Can you work these out from the model? Positions are in its coordinate system, mm. Face numbers are marked on the shaded views. A direction names the side the tool comes from. Coordinates: 2 decimals unless noted, no trailing zeros. Order: outer loops, then holes, each group sorted by start corner. A loop starts at its lowest first (then second) coordinate and runs counter-clockwise, first axis right, second up. Notation, with made-up numbers: (86, -19) -> (107, -19) arc R9 ccw to (107, -7) -> close; hole circle Ø7 at (-3, 55.5). An arc over 180 degrees is marked (long way). Use a Markdown table: item, result. Add a question column.
1. We'd pull the mould along X, two halves only. Please class the marked faces 5, 6 and 7: pulls with the +X half, pulls with the -X half, needs draft (parallel to the pull), parting line crosses it, or undercut.
2. Suppose I cut it at D-D, the plane y = -7. List the corners of the cut face in (x, z) for me.
3. For pin 1 Ø5 at (x, z) = (-16.5, 24) entering from +Y; pin 2 Ø4 at (x, y) = (-22, -3.5) entering from -Z; pin 3 Ø3 at (y, z) = (-3.5, 19.5) entering from +X; pin 4 Ø2 at (x, z) = (-2.5, 21) entering from -Y, each with a flat end and sliding along its axis, tell me the tip position at first contact or that it passes through.
4. Suppose I cut it at C-C, the plane y = -2.25. List the corners of the cut face in (x, z) for me, then the cut area to 3 significant figures.
5. Suppose I cut it at B-B, the plane x = -17.5. List the corners of the cut face in (y, z) for me.
6. If I drill on line 1 along X through (y, z) = (-1.5, 17); line 2 along Y through (x, z) = (-23.5, 23.25); line 3 along X through (y, z) = (-7, 25.25), over which ranges is the centre line in solid material (lowest first)? Write a range as from..to.
7. For the marked faces 1, 2, 3 and 4, which set-ups out of +Z, -Z, +X, -X, +Y, -Y let a thin tool reach every point of the face, with its end or its side?
8. Suppose I cut it at A-A, the plane z = 27.75. List the corners of the cut face in (x, y) for me, then the cut area to 3 significant figures.
```python
from build123d import *

# Parameters (mm, degrees)
SKETCH1_W           = 35
SKETCH1_H           = 175
BOSS_EXTRUDE1_DEPTH = 7.5
SKETCH2_W           = 25
SKETCH2_H           = 6.5
CUT_EXTRUDE1_DEPTH  = 179.623206779
CUT_EXTRUDE2_DEPTH  = 179.623206779
SKETCH4_W           = 4
SKETCH4_H           = 6.5
CUT_EXTRUDE3_DEPTH  = 179.623206779
SKETCH5_W           = 4
SKETCH5_H           = 6.5
CUT_EXTRUDE4_DEPTH  = 179.623206779
CUT_EXTRUDE5_DEPTH  = 179.623206779
CUT_EXTRUDE6_DEPTH  = 179.584013842
CUT_EXTRUDE7_DEPTH  = 179.584013842
CUT_EXTRUDE8_DEPTH  = 179.584013842
CUT_EXTRUDE9_DEPTH  = 179.584013842
CUT_EXTRUDE10_DEPTH = 179.584013842
CUT_EXTRUDE11_DEPTH = 179.623206779
SKETCH13_W          = 54.072725276
SKETCH13_H          = 30.837150003
CUT_EXTRUDE12_DEPTH = 15
SKETCH14_W          = 49.0024185
SKETCH14_H          = 27.053522809
CUT_EXTRUDE13_DEPTH = 142


with BuildPart() as part:
    # Sketch1 → Boss-Extrude1 (new body)
    with BuildSketch(Plane(origin=(0, 0, 0), x_dir=(1, 0, 0), z_dir=(0, 1, 0))):
        with Locations((-17.5, -87.5)):
            Rectangle(SKETCH1_W, SKETCH1_H)
    extrude(amount=-BOSS_EXTRUDE1_DEPTH)

    # Sketch2 → Cut-Extrude1 (cut, through all)
    with BuildSketch(Plane(origin=(0, 0, 0), x_dir=(-1, 0, 0), z_dir=(0, 0, -1))):
        with Locations((17.5, -3.25)):
            Rectangle(SKETCH2_W, SKETCH2_H)
    extrude(amount=-CUT_EXTRUDE1_DEPTH, mode=Mode.SUBTRACT)

    # Sketch3 → Cut-Extrude2 (cut, through all)
    with BuildSketch(Plane.XZ.offset(7.5)):
        with BuildLine():
            Line((-20.6, 0), (-14.4, 0))
            Line((-14.4, 0), (-14.4, 3.4))
            ThreePointArc((-14.4, 3.4), (-17.5, 6.5), (-20.6, 3.4))
            Line((-20.6, 3.4), (-20.6, 0))
        make_face()
    extrude(amount=-CUT_EXTRUDE2_DEPTH, mode=Mode.SUBTRACT)

    # Sketch4 → Cut-Extrude3 (cut, through all)
    with BuildSketch(Plane(origin=(0, 0, 0), x_dir=(-1, 0, 0), z_dir=(0, 0, -1))):
        with Locations((33, -4.25)):
            Rectangle(SKETCH4_W, SKETCH4_H)
    extrude(amount=-CUT_EXTRUDE3_DEPTH, mode=Mode.SUBTRACT)

    # Sketch5 → Cut-Extrude4 (cut, through all)
    with BuildSketch(Plane(origin=(0, 0, 0), x_dir=(-1, 0, 0), z_dir=(0, 0, -1))):
        with Locations((2, -4.25)):
            Rectangle(SKETCH5_W, SKETCH5_H)
    extrude(amount=-CUT_EXTRUDE4_DEPTH, mode=Mode.SUBTRACT)

    # Sketch6 → Cut-Extrude5 (cut, through all)
    with BuildSketch(Plane.XZ.offset(7.5)):
        with BuildLine():
            Line((-14.4, 175), (-20.6, 175))
            Line((-20.6, 175), (-20.6, 169.6))
            ThreePointArc((-20.6, 169.6), (-17.5, 166.5), (-14.4, 169.6))
            Line((-14.4, 169.6), (-14.4, 175))
        make_face()
    extrude(amount=-CUT_EXTRUDE5_DEPTH, mode=Mode.SUBTRACT)

    # Sketch7 → Cut-Extrude6 (cut, through all)
    with BuildSketch(Plane(origin=(0, -6.5, 0), x_dir=(-1, 0, 0), z_dir=(0, 1, 0))):
        with BuildLine():
            Line((14.4, 103.4), (14.4, 94.6))
            ThreePointArc((14.4, 94.6), (17.5, 91.5), (20.6, 94.6))
            Line((20.6, 94.6), (20.6, 103.4))
            ThreePointArc((20.6, 103.4), (17.5, 106.5), (14.4, 103.4))
        make_face()
    extrude(amount=-CUT_EXTRUDE6_DEPTH, mode=Mode.SUBTRACT)

    # Sketch8 → Cut-Extrude7 (cut, through all)
    with BuildSketch(Plane(origin=(0, -6.5, 0), x_dir=(-1, 0, 0), z_dir=(0, 1, 0))):
        with BuildLine():
            Line((14.4, 78.4), (14.4, 69.6))
            ThreePointArc((14.4, 69.6), (17.5, 66.5), (20.6, 69.6))
            Line((20.6, 69.6), (20.6, 78.4))
            ThreePointArc((20.6, 78.4), (17.5, 81.5), (14.4, 78.4))
        make_face()
    extrude(amount=-CUT_EXTRUDE7_DEPTH, mode=Mode.SUBTRACT)

    # Sketch9 → Cut-Extrude8 (cut, through all)
    with BuildSketch(Plane(origin=(0, -6.5, 0), x_dir=(-1, 0, 0), z_dir=(0, 1, 0))):
        with BuildLine():
            Line((14.4, 28.4), (14.4, 19.6))
            ThreePointArc((14.4, 19.6), (17.5, 16.5), (20.6, 19.6))
            Line((20.6, 19.6), (20.6, 28.4))
            ThreePointArc((20.6, 28.4), (17.5, 31.5), (14.4, 28.4))
        make_face()
    extrude(amount=-CUT_EXTRUDE8_DEPTH, mode=Mode.SUBTRACT)

    # Sketch10 → Cut-Extrude9 (cut, through all)
    with BuildSketch(Plane(origin=(0, -6.5, 0), x_dir=(-1, 0, 0), z_dir=(0, 1, 0))):
        with BuildLine():
            Line((14.4, 153.4), (14.4, 144.6))
            ThreePointArc((14.4, 144.6), (17.5, 141.5), (20.6, 144.6))
            Line((20.6, 144.6), (20.6, 153.4))
            ThreePointArc((20.6, 153.4), (17.5, 156.5), (14.4, 153.4))
        make_face()
    extrude(amount=-CUT_EXTRUDE9_DEPTH, mode=Mode.SUBTRACT)

    # Sketch11 → Cut-Extrude10 (cut, through all)
    with BuildSketch(Plane(origin=(0, -6.5, 0), x_dir=(-1, 0, 0), z_dir=(0, 1, 0))):
        with BuildLine():
            Line((14.4, 128.4), (14.4, 119.6))
            ThreePointArc((14.4, 119.6), (17.5, 116.5), (20.6, 119.6))
            Line((20.6, 119.6), (20.6, 128.4))
            ThreePointArc((20.6, 128.4), (17.5, 131.5), (14.4, 128.4))
        make_face()
    extrude(amount=-CUT_EXTRUDE10_DEPTH, mode=Mode.SUBTRACT)

    # Sketch12 → Cut-Extrude11 (cut, through all)
    with BuildSketch(Plane.XZ.offset(7.5)):
        with BuildLine():
            Line((-20.6, 53.4), (-20.6, 44.6))
            ThreePointArc((-20.6, 44.6), (-17.5, 41.5), (-14.4, 44.6))
            Line((-14.4, 44.6), (-14.4, 53.4))
            ThreePointArc((-14.4, 53.4), (-17.5, 56.5), (-20.6, 53.4))
        make_face()
    extrude(amount=-CUT_EXTRUDE11_DEPTH, mode=Mode.SUBTRACT)

    # Sketch13 → Cut-Extrude12 (cut)
    with BuildSketch(Plane(origin=(0, 0, 0), x_dir=(-1, 0, 0), z_dir=(0, 0, -1))):
        with Locations((12.505255608, -4.443731482)):
            Rectangle(SKETCH13_W, SKETCH13_H)
    extrude(amount=-CUT_EXTRUDE12_DEPTH, mode=Mode.SUBTRACT)

    # Sketch14 → Cut-Extrude13 (cut)
    with BuildSketch(Plane.XY.offset(175)):
        with Locations((-15.887003793, 1.102839907)):
            Rectangle(SKETCH14_W, SKETCH14_H)
    extrude(amount=-CUT_EXTRUDE13_DEPTH, mode=Mode.SUBTRACT)


solid = part.part
```
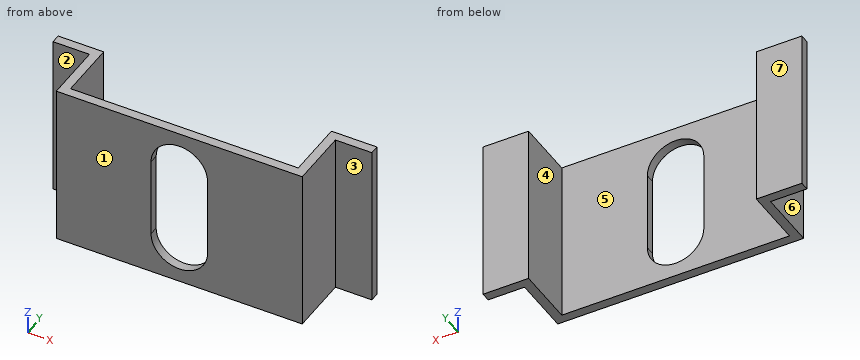
Worked out:
| question | item | result |
|---|---|---|
| 1 | face 5 | undercut |
| 1 | face 6 | pulls with the -X half |
| 1 | face 7 | needs draft |
| 2 | outline | (-31, 15) -> (-4, 15) -> (-4, 33) -> (-31, 33) -> close; hole (-20.6, 19.6) arc R3.1 ccw to (-14.4, 19.6) -> (-14.4, 28.4) arc R3.1 ccw to (-20.6, 28.4) -> close |
| 3 | pin 1 | stops at y = -6.5 |
| 3 | pin 2 | passes through |
| 3 | pin 3 | stops at x = -4 |
| 3 | pin 4 | stops at y = -1 |
| 4 | outline | (-31, 15) -> (-30, 15) -> (-30, 33) -> (-31, 33) -> close; (-5, 15) -> (-4, 15) -> (-4, 33) -> (-5, 33) -> close |
| 4 | area | 36.0 mm² |
| 5 | outline | (-7.5, 15) -> (-6.5, 15) -> (-6.5, 16.5) -> (-7.5, 16.5) -> close; (-7.5, 31.5) -> (-6.5, 31.5) -> (-6.5, 33) -> (-7.5, 33) -> close |
| 6 | line 1 | x = -31..-30, -5..-4 |
| 6 | line 2 | y = -7.5..-6.5 |
| 6 | line 3 | x = -31..-20.6, -14.4..-4 |
| 7 | face 1 | +Z, -Z, +X, -X, -Y |
| 7 | face 2 | +Z, -Z, -X, -Y |
| 7 | face 3 | +Z, -Z, +X, -Y |
| 7 | face 4 | +Z, -Z, +Y |
| 8 | outline | (-35, -1) -> (-31, -1) -> (-31, -7.5) -> (-20.6, -7.5) -> (-20.6, -6.5) -> (-30, -6.5) -> (-30, 0) -> (-35, 0) -> close; (-14.4, -7.5) -> (-4, -7.5) -> (-4, -1) -> (0, -1) -> (0, 0) -> (-5, 0) -> (-5, -6.5) -> (-14.4, -6.5) -> close |
| 8 | area | 41.8 mm² |
